Check sheet for the modelled part. Datum: model origin and axes. Units: mm. Face numbers are marked on the shaded views. A direction names the side the tool comes from. Give positions to 0.01 mm unless a question says otherwise; leave off trailing zeros. Loops run counter-clockwise (first coordinate to the right, second up) from the corner with the lowest first, then second, coordinate; pieces in that order, holes last. Notation, with made-up numbers: M 10.25,-30.75 L 44.25,-30.75 A23 ccw 44.25,-22.75 Z; hole C -18,79.5 d8. An arc over 180 degrees is marked long. Write each question's results on one line, items separated by ' | '. Start each with the question number.
1. Sectioned sample at D-D on y = -40. Record the cut outline in (x, z).
2. Tool access check on the marked faces 1, 2 and 3. Record the directions out of +Z, -Z, +X, -X, +Y, -Y that give a thin tool (end or side, any length) a straight path to the whole face; none if there is none.
3. Material ranges on line 1 along Z through (x, y) = (19.5, -1.9); line 2 along X through (y, z) = (-2.2, 4.5); line 3 along Y through (x, z) = (28.7, 25), recorded low to high.
4. Sectioned sample at A-A on x = 16.5. Record the cut outline in (y, z), and give its area (3 significant figures).
5. Sectioned sample at B-B on z = 15. Record the cut outline in (x, y), and give its area (3 significant figures).
6. Sectioned sample at C-C on x = 19.5. Record the cut outline in (y, z).
7. Go/stop test with a flat-tipped pin: pin 1 (4.5 mm diameter, centred on x = 19.5, z = 35.5, fed in from -Y). Record where the tip stops, or that it passes through.
```python
from build123d import *

# Parameters (mm, degrees)
EXTRUDE_1_DEPTH     = 40
SKETCH_2_R          = 1.65
SKETCH_2_W          = 27
SKETCH_2_H          = 22
CUT_EXTRUDE_2_DEPTH = 10
SKETCH_3_R          = 2
SKETCH_3_W          = 22
SKETCH_3_H          = 41
CUT_EXTRUDE_3_DEPTH = 10


with BuildPart() as part:
    # 草图1 → 凸台-拉伸1 (new body)
    with BuildSketch(Plane.XY):
        Polygon((0, 0), (30, 0), (30, -60), (27, -60), (27, -3), (0, -3), align=None)
    extrude(amount=EXTRUDE_1_DEPTH)

    # 草图2 → 切除-拉伸2 (cut)
    with BuildSketch(Plane(origin=(0, 0, 0), x_dir=(1, 0, 0), z_dir=(0, 1, 0))):
        with Locations((7.5, -4.5)):
            Circle(SKETCH_2_R)
        with Locations((19.5, -4.5)):
            Circle(SKETCH_2_R)
        with Locations((19.5, -35.5)):
            Circle(SKETCH_2_R)
        with Locations((7.5, -35.5)):
            Circle(SKETCH_2_R)
        with Locations((13.5, -20)):
            Rectangle(SKETCH_2_W, SKETCH_2_H)
    extrude(amount=-CUT_EXTRUDE_2_DEPTH, mode=Mode.SUBTRACT)

    # 草图3 → 切除-拉伸3 (cut)
    with BuildSketch(Plane(origin=(30, 0, 0), x_dir=(0, 0, -1), z_dir=(1, 0, 0))):
        with Locations((-25, -5)):
            Circle(SKETCH_3_R)
        with Locations((-15, -5)):
            Circle(SKETCH_3_R)
        with Locations((-15, -55)):
            Circle(SKETCH_3_R)
        with Locations((-25, -55)):
            Circle(SKETCH_3_R)
        with Locations((-20, -30)):
            Rectangle(SKETCH_3_W, SKETCH_3_H)
    extrude(amount=-CUT_EXTRUDE_3_DEPTH, mode=Mode.SUBTRACT)


solid = part.part
```
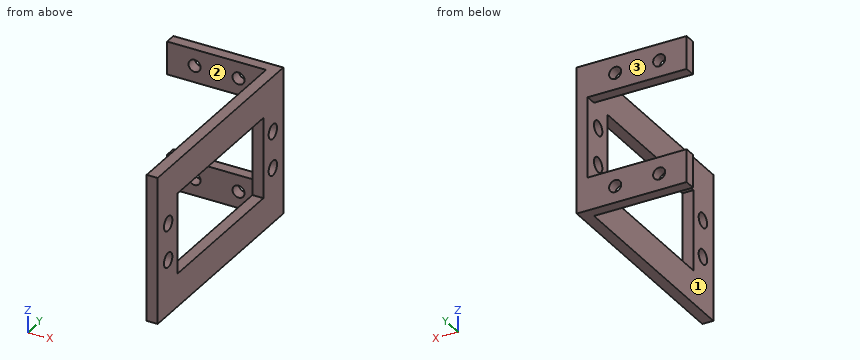
Output values:
1) outline: M 27,0 L 30,0 L 30,9 L 27,9 Z; M 27,31 L 30,31 L 30,40 L 27,40 Z
2) face 1: -X, -Y | face 2: +Z, -Z, -X, -Y | face 3: +Z, -Z, +X, -X, +Y
3) line 1: 0 to 2.85, 6.15 to 9, 31 to 33.85, 37.15 to 40 | line 2: 0 to 5.85, 9.15 to 17.85, 21.15 to 30 | line 3: -60 to -57, -53 to -50.5, -9.5 to -7, -3 to 0
4) outline: M -3,0 L 0,0 L 0,9 L -3,9 Z; M -3,31 L 0,31 L 0,40 L -3,40 Z | area: 54.0 mm2
5) outline: M 27,-60 L 30,-60 L 30,-57 L 27,-57 Z; M 27,-53 L 30,-53 L 30,-50.5 L 27,-50.5 Z; M 27,-9.5 L 30,-9.5 L 30,-7 L 27,-7 Z; M 27,-3 L 30,-3 L 30,0 L 27,0 Z | area: 33.0 mm2
6) outline: M -3,0 L 0,0 L 0,2.85 L -3,2.85 Z; M -3,6.15 L 0,6.15 L 0,9 L -3,9 Z; M -3,31 L 0,31 L 0,33.85 L -3,33.85 Z; M -3,37.15 L 0,37.15 L 0,40 L -3,40 Z
7) pin 1: y = -3
